from build123d import *

# Parameters (mm, degrees)
EXTRUDE_1_DEPTH = 10
SKETCH_2_R      = 0.8
EXTRUDE_2_DEPTH = 0.5
EXTRUDE_3_DEPTH = 6.7
EXTRUDE_4_DEPTH = 3
SKETCH_5_R      = 1.6
EXTRUDE_5_DEPTH = 3


with BuildPart() as part:
    # 草图1 → 凸台-拉伸1 (new body)
    with BuildSketch(Plane(origin=(0, 0, 0), x_dir=(1, 0, 0), z_dir=(0, 1, 0))):
        with BuildLine():
            Line((-7, -4), (7, -4))
            ThreePointArc((7, -4), (7.707106781, -3.707106781), (8, -3))
            Line((8, -3), (8, 3))
            ThreePointArc((8, 3), (7.707106781, 3.707106781), (7, 4))
            Line((7, 4), (-7, 4))
            ThreePointArc((-7, 4), (-7.707106781, 3.707106781), (-8, 3))
            Line((-8, 3), (-8, -3))
            ThreePointArc((-8, -3), (-7.707106781, -3.707106781), (-7, -4))
        make_face()
    extrude(amount=EXTRUDE_1_DEPTH)

    # 草图2 → 凸台-拉伸2 (add)
    with BuildSketch(Plane(origin=(0, 10, 0), x_dir=(1, 0, 0), z_dir=(0, 1, 0))):
        with BuildLine():
            Line((-10, -4), (10, -4))
            ThreePointArc((10, -4), (12.5, 0), (10, 4))
            Line((10, 4), (-10, 4))
            ThreePointArc((-10, 4), (-12.5, 0), (-10, -4))
        make_face()
        with Locations(Location((-10, 0, 0), (0, 0, 270))):
            Circle(SKETCH_2_R, mode=Mode.SUBTRACT)
        with Locations(Location((10, 0, 0), (0, 0, 90))):
            Circle(SKETCH_2_R, mode=Mode.SUBTRACT)
    extrude(amount=EXTRUDE_2_DEPTH)

    # 草图3 → 凸台-拉伸3 (add)
    with BuildSketch(Plane(origin=(0, 10.5, 0), x_dir=(1, 0, 0), z_dir=(0, 1, 0))):
        with BuildLine():
            Line((7, 4), (-7, 4))
            ThreePointArc((-7, 4), (-7.707106781, 3.707106781), (-8, 3))
            Line((-8, 3), (-8, -3))
            ThreePointArc((-8, -3), (-7.707106781, -3.707106781), (-7, -4))
            Line((-7, -4), (7, -4))
            ThreePointArc((7, -4), (7.707106781, -3.707106781), (8, -3))
            Line((8, -3), (8, 3))
            ThreePointArc((8, 3), (7.707106781, 3.707106781), (7, 4))
        make_face()
    extrude(amount=EXTRUDE_3_DEPTH)

    # 草图4 → 凸台-拉伸4 (add)
    with BuildSketch(Plane(origin=(0, 17.2, 0), x_dir=(1, 0, 0), z_dir=(0, 1, 0))):
        with BuildLine():
            Line((-1.119183588, 0.8), (0.080816412, 0.8))
            ThreePointArc((0.080816412, 0.8), (8, 0), (0.080816412, -0.8))
            Line((0.080816412, -0.8), (-1.119183588, -0.8))
            ThreePointArc((-1.119183588, -0.8), (-1.919183588, 0), (-1.119183588, 0.8))
        make_face()
    extrude(amount=EXTRUDE_4_DEPTH)

    # 草图5 → 凸台-拉伸5 (add)
    with BuildSketch(Plane(origin=(0, 20.2, 0), x_dir=(1, 0, 0), z_dir=(0, 1, 0))):
        with Locations(Location((4, 0, 0), (0, 0, 270))):
            Circle(SKETCH_5_R)
    extrude(amount=EXTRUDE_5_DEPTH)


solid = part.part
Part model, mm, in its own coordinate system. A direction names the side the tool comes from. Give positions to 0.01 mm unless a question says otherwise; leave off trailing zeros. Write each loop counter-clockwise with the first axis right and the second up, starting at its lowest first coordinate (ties: lowest second). Pieces come first, ordered by that corner, then holes.
1) Which spindle directions (+Z, -Z, +X, -X, +Y, -Y) get a long thin tool onto all of the face, cutting with end or side? Do faces 1 (the face through (8, 5, 0)), 2 (the face through (-7.699, 13.803, -3.715)), 3 (the face through (4, 20.2, -2)), 4 (the face through (7.699, 13.803, 3.715)), 5 (the face through (7.715, 13.803, -3.699)). Say none if no direction does.
Resolved:
face 1: +Z, -Z, +X, -Y
face 2: -Z, -X, +Y
face 3: +Y
face 4: +Z, +X, +Y
face 5: -Z, +X, +Y
2) Pin check, flat tips, straight feed: pin 1 (1.8 mm diameter, centred on x = -10, z = 0, fed in from -Y); pin 2 (3 mm diameter, centred on y = 13, z = -0.5, fed in from +X); pin 3 (3 mm diameter, centred on x = 6, z = 2.5, fed in from +Y); pin 4 (1 mm diameter, centred on x = -4, y = 19.5, fed in from +Z). Stop position of each tip, or through.
Resolved:
pin 1: stops at y = 10
pin 2: stops at x = 8
pin 3: stops at y = 20.2
pin 4: passes through
3) Probe L1, parallel to X at y = 10.3, z = 0; L2, parallel to X at y = 12.5, z = 2.25; L3, parallel to Z at x = 10, y = 10.2. List the from-to ranges inside material, lowest first.
Resolved:
L1: x = -12.5 to -10.8, -9.2 to 9.2, 10.8 to 12.5
L2: x = -8 to 8
L3: z = -4 to -0.8, 0.8 to 4
4) Cut at D-D on z = 2.5. Write the cut outline in (x, y), then the cut area to 3 significant figures.
Resolved:
outline: (-11.73, 10) - (-8, 10) - (-8, 0) - (8, 0) - (8, 10) - (11.73, 10) - (11.73, 10.5) - (8, 10.5) - (8, 17.2) - (7.12, 17.2) - (7.12, 20.2) - (0.88, 20.2) - (0.88, 17.2) - (-8, 17.2) - (-8, 10.5) - (-11.73, 10.5) - close
area: 298 mm2
5) Cut at C-C on x = 10.5. Write the cut outline in (y, z).
Resolved:
outline: (10, -3.71) - (10.5, -3.71) - (10.5, -0.62) - (10, -0.62) - close; (10, 0.62) - (10.5, 0.62) - (10.5, 3.71) - (10, 3.71) - close
6) Two-plate mould, pull along X, no slides. Class faces 6 (the face through (-8, 5, 0)), 7 (the face through (-9.207, 10.246, -0.104)), 8 (the face through (2.44, 21.68, -0.35)): released by +X, released by -X, zero draft, split by the parting line, or undercut.
Resolved:
face 6: released by -X
face 7: undercut
face 8: split by the parting line
7) Cut at A-A on x = -0.5. Write the cut outline in (y, z), then the cut area to 3 significant figures.
Resolved:
outline: (0, -4) - (17.2, -4) - (17.2, -0.8) - (20.2, -0.8) - (20.2, 0.8) - (17.2, 0.8) - (17.2, 4) - (0, 4) - close
area: 142 mm2
8) Cut at B-B on y = 9.25. Write the cut outline in (x, z), then the cut area to 3 significant figures.
Resolved:
outline: (-8, -3) arc R1 ccw to (-7, -4) - (7, -4) arc R1 ccw to (8, -3) - (8, 3) arc R1 ccw to (7, 4) - (-7, 4) arc R1 ccw to (-8, 3) - close
area: 127 mm2
